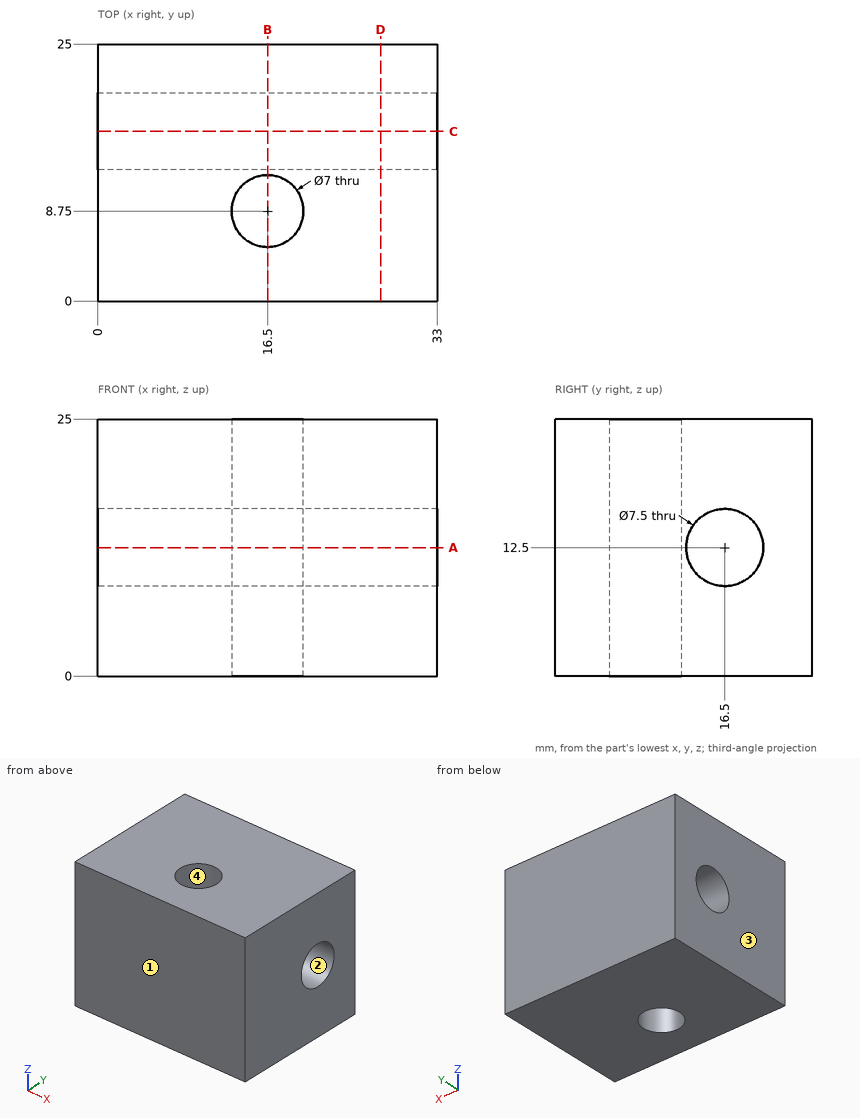
For this review, use the dimensioned drawing (mm, ordinates from the lowest corner) and the shaded views. Round coordinates to 2 decimals unless told otherwise and drop trailing zeros. Write each loop counter-clockwise with the first axis right and the second up, starting at its lowest first coordinate (ties: lowest second). Pieces come first, ordered by that corner, then holes. Notation, with made-up numbers: (48, -13) -> (88, -13) arc R27 ccw to (88, 8) -> close; hole circle Ø5 at (42, -4). An arc over 180 degrees is marked (long way). Answer in a Markdown table with one row per item.
Q1. To check wall thickness, follow L1, parallel to X at y = 8.75, z = 13.5; L2, parallel to Z at x = 7, y = 16.5; L3, parallel to Y at x = 24, z = 12.5. State the ranges of each line that lie inside material, in increasing order. Write a range as [from, to].
The answers:
| item | result |
|---|---|
| L1 | [0, 13], [20, 33] |
| L2 | [0, 8.75], [16.25, 25] |
| L3 | [0, 12.75], [20.25, 25] |
Q2. Take a section at C-C, the plane y = 16.5. State the section outline as (x, z) points, then the cut area to 4 significant figures.
The answers:
| item | result |
|---|---|
| outline | (0, 0) -> (33, 0) -> (33, 8.75) -> (0, 8.75) -> close; (0, 16.25) -> (33, 16.25) -> (33, 25) -> (0, 25) -> close |
| area | 577.5 mm² |
Q3. Draft analysis for pull direction Y (two halves, no side actions). For the marked faces 1, 2, 3 and 4, state which applies: +Y half, -Y half, draft (parallel to the pull), parting line (faces both ways), or undercut.
The answers:
| item | result |
|---|---|
| face 1 | -Y half |
| face 2 | undercut |
| face 3 | draft |
| face 4 | undercut |
Q4. Take a section at A-A, the plane z = 12.5. State the section outline as (x, y) points, then the cut area to 3 significant figures.
The answers:
| item | result |
|---|---|
| outline | (0, 0) -> (33, 0) -> (33, 12.75) -> (0, 12.75) -> close; (0, 20.25) -> (33, 20.25) -> (33, 25) -> (0, 25) -> close; hole circle Ø7 at (16.5, 8.75) |
| area | 539 mm² |
Q5. Clearance check with a flat-ended pin moving along its axis: pin 1 Ø4 at (x, y) = (16.5, 8.75) entering from -Z. State where the tip first meets the part, or that it passes through.
The answers:
| item | result |
|---|---|
| pin 1 | through |
Q6. Take a section at D-D, the plane x = 27.5. State the section outline as (y, z) points, then the cut area to 3 significant figures.
The answers:
| item | result |
|---|---|
| outline | (0, 0) -> (25, 0) -> (25, 25) -> (0, 25) -> close; hole circle Ø7.5 at (16.5, 12.5) |
| area | 581 mm² |
Q7. Take a section at B-B, the plane x = 16.5. State the section outline as (y, z) points, then the cut area to 3 significant figures.
The answers:
| item | result |
|---|---|
| outline | (0, 0) -> (5.25, 0) -> (5.25, 25) -> (0, 25) -> close; (12.25, 0) -> (25, 0) -> (25, 25) -> (12.25, 25) -> close; hole circle Ø7.5 at (16.5, 12.5) |
| area | 406 mm² |
